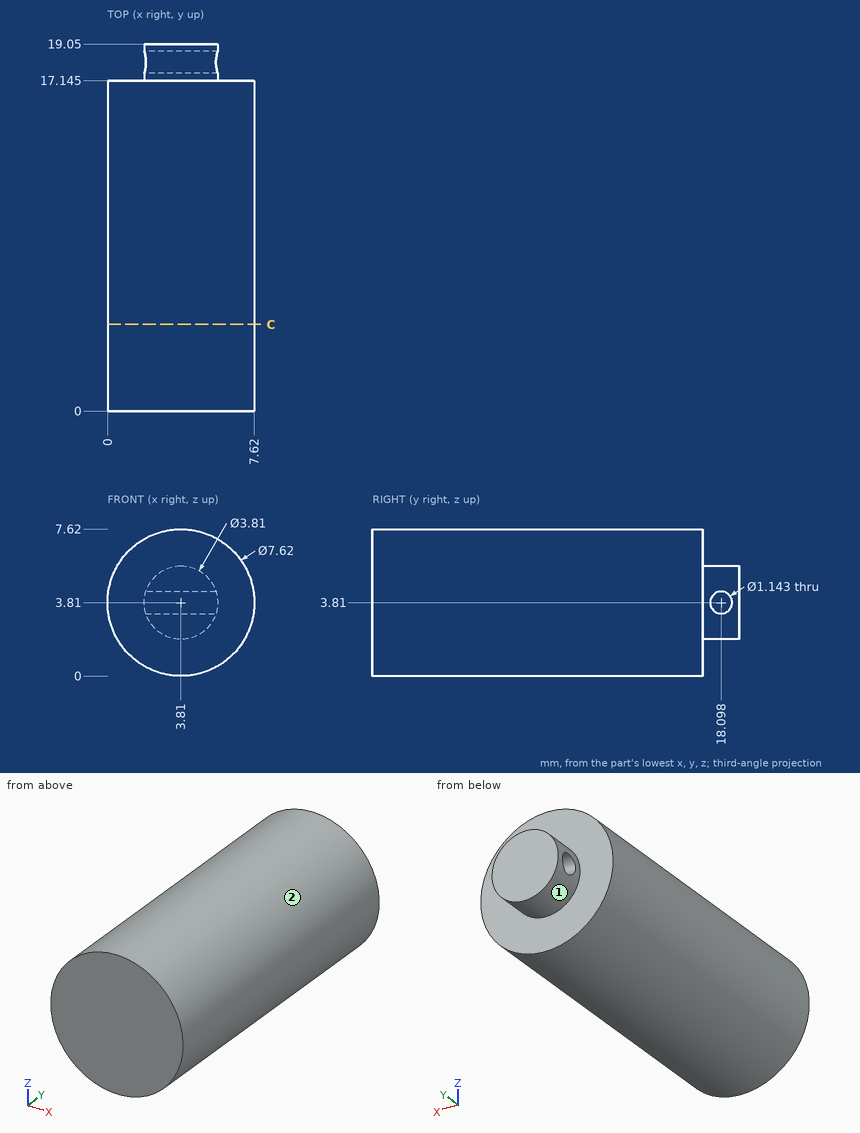
Geometry check sheet. Reference: drawing and pictorial views, mm from the part's lowest x, y, z. A direction names the side the tool comes from. Coordinates: 2 decimals unless noted, no trailing zeros. Write each loop counter-clockwise with the first axis right and the second up, starting at its lowest first coordinate (ties: lowest second). Pieces come first, ordered by that corner, then holes.
Item 1: Cross-section at C-C on y = 4.5. Record the boundary of the cut face in (x, z), then the cut area to 3 significant figures.
Numbers:
outline: circle Ø7.62 at (3.81, 3.81)
area: 45.6 mm2
Item 2: Access from +Z, -Z, +X, -X, +Y, -Y to the whole of each face (thin tool, end or side, straight path). Record for the marked faces 1 and 2.
Numbers:
face 1: +Y
face 2: +Y, -Y
Item 3: Depth check by flat-ended pin: pin 1 Ø1 at (y, z) = (11, 4) entering from -X; pin 2 Ø1.5 at (y, z) = (9, 6) entering from -X; pin 3 Ø1.3 at (y, z) = (18.1, 3.81) entering from +X (1 decimal). Enter the tip coordinate at first touch or a pass-through.
Numbers:
pin 1: stops at x = 0
pin 2: stops at x = 0.28
pin 3: stops at x = 5.7
Item 4: Scan lines: probe 1 along Y at (x, z) = (5.75, 6.25) (1 decimal); probe 2 along X at (y, z) = (8, 4.5); probe 3 along Z at (x, y) = (2, 2.25). Record each from-to range of solid material in increasing order.
Numbers:
probe 1: y = 0 to 17.1
probe 2: x = 0.06 to 7.56
probe 3: z = 0.46 to 7.16
